Check sheet for the modelled part. Datum: model origin and axes. Units: mm. Round coordinates to 2 decimals unless told otherwise and drop trailing zeros. Write each loop counter-clockwise with the first axis right and the second up, starting at its lowest first coordinate (ties: lowest second). Pieces come first, ordered by that corner, then holes. Notation, with made-up numbers: (19, 51) -> (47, 51) arc R22 ccw to (47, 74) -> close; hole circle Ø6 at (8, -21). An arc over 180 degrees is marked (long way). Put each result on its own line as item: value. Start each with the question number.
from build123d import *

# Parameters (mm, degrees)
SKETCH1_R           = 0.635
BOSS_EXTRUDE1_DEPTH = 3.175


with BuildPart() as part:
    # Sketch1 → Boss-Extrude1 (new body)
    with BuildSketch(Plane.XY):
        Polygon((169.876910838, 126.650867177), (1.5875, 125.794558197), (1.5875, 139.257710065), (169.000191682, 139.858675371), align=None)
        with Locations((157.892850269, 129.235572603)):
            Circle(SKETCH1_R, mode=Mode.SUBTRACT)
        with Locations((14.087503577, 132.842415442)):
            Circle(SKETCH1_R, mode=Mode.SUBTRACT)
        with Locations((7.163696951, 133.477415442)):
            Circle(SKETCH1_R, mode=Mode.SUBTRACT)
    extrude(amount=-BOSS_EXTRUDE1_DEPTH)


solid = part.part
1. Section check B-B, the plane x = 49.5. Enter the section's corners in (y, z) (3 decimals), then the cut area to 3 significant figures.
2. Gauge pin test, flat ends, axial feed: P1, Ø1, axis at x = 7.16, y = 133.48, coming from the +Z side; P2, Ø1, axis at x = 122.5, z = -2.5, coming from the +Y side. Record the tip position at first contact, or that the pin passes through.
3. Section check C-C, the plane x = 76. Enter the section's corners in (y, z) (3 decimals).
4. Material ranges on L1, parallel to X at y = 134, z = -1.45; L2, parallel to X at y = 133.75, z = -1.2; L3, parallel to Y at x = 116.5, z = -2.4, recorded low to high. Write a range as [from, to].
5. Section check A-A, the plane z = -1.35. Enter the section's corners in (x, y) (1 decimal).
Reply:
1. outline: (126.038, -3.175) -> (139.43, -3.175) -> (139.43, 0) -> (126.038, 0) -> close
1. area: 42.5 mm2
2. P1: passes through
2. P2: stops at y = 139.69
3. outline: (126.173, -3.175) -> (139.525, -3.175) -> (139.525, 0) -> (126.173, 0) -> close
4. L1: x = [1.59, 6.8], [7.52, 169.39]
4. L2: x = [1.59, 6.59], [7.74, 169.41]
4. L3: y = [126.38, 139.67]
5. outline: (1.6, 125.8) -> (169.9, 126.7) -> (169, 139.9) -> (1.6, 139.3) -> close; hole circle Ø1.3 at (7.2, 133.5); hole circle Ø1.3 at (14.1, 132.8); hole circle Ø1.3 at (157.9, 129.2)
